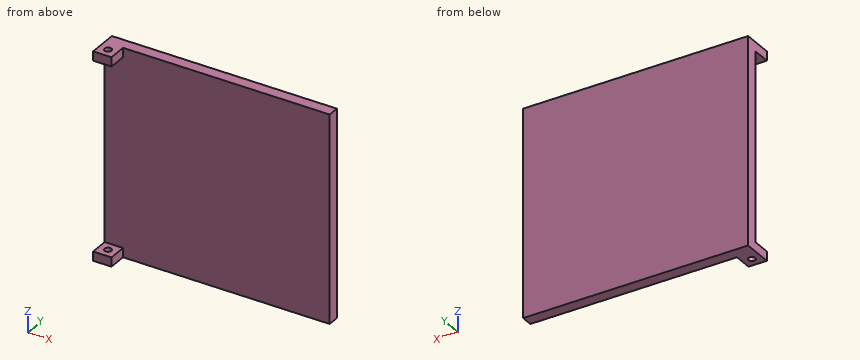
from build123d import *

# Parameters (mm, degrees)
SKETCH_1_W          = 39.2
SKETCH_1_H          = 36
EXTRUDE_1_DEPTH     = 2
SKETCH_7_W          = 3.2
SKETCH_7_H          = 1.6
EXTRUDE_3_DEPTH     = 3.2
CUT_EXTRUDE_START   = -36
SKETCH_8_R          = 0.6
CUT_EXTRUDE_2_DEPTH = 36


with BuildPart() as part:
    # Эскиз1 → Бобышка-Вытянуть1 (new body)
    with BuildSketch(Plane(origin=(0, 0, 0), x_dir=(1, 0, 0), z_dir=(0, 1, 0))):
        Rectangle(SKETCH_1_W, SKETCH_1_H)
    extrude(amount=EXTRUDE_1_DEPTH)

    # Эскиз7 → Бобышка-Вытянуть3 (add)
    with BuildSketch(Plane.XZ):
        with Locations((-18, -17.2)):
            Rectangle(SKETCH_7_W, SKETCH_7_H)
        with Locations((-18, 17.2)):
            Rectangle(SKETCH_7_W, SKETCH_7_H)
    extrude(amount=EXTRUDE_3_DEPTH)

    # Эскиз8 → Вырез-Вытянуть2 (cut)
    with BuildSketch(Plane(origin=(0, 0, -18), x_dir=(-1, 0, 0), z_dir=(0, 0, -1)).offset(CUT_EXTRUDE_START)):
        with Locations((18, -1.6)):
            Circle(SKETCH_8_R)
    extrude(amount=CUT_EXTRUDE_2_DEPTH, mode=Mode.SUBTRACT)


solid = part.part
CAD build for the part. Positions are in the model's coordinates, mm. Round coordinates to 2 decimals unless told otherwise and drop trailing zeros. Write each loop counter-clockwise with the first axis right and the second up, starting at its lowest first coordinate (ties: lowest second). Pieces come first, ordered by that corner, then holes. Notation, with made-up numbers: M 54,13 L 74,13 A20 ccw 74,24 Z; hole C 9,58 d1. An arc over 180 degrees is marked long. Put each result on its own line as item: value. Start each with the question number.
1) Pin check, flat tips, straight feed: pin 1 Ø3 at (x, z) = (6, 7.5) entering from -Y; pin 2 Ø1.8 at (y, z) = (-2, 17) entering from +X; pin 3 Ø1.1 at (x, y) = (-18, -1.6) entering from +Z; pin 4 Ø1.9 at (x, y) = (-18, -1.6) entering from +Z. Stop position of each tip, or through.
2) Saw through at B-B, the plane y = -1.6. Write the cut outline in (x, z).
3) Drill centre lines: probe 1 along Y at (x, z) = (-18, 17); probe 2 along Y at (x, z) = (3, -3); probe 3 along X at (y, z) = (-1.6, 16.9). Where is each one in solid material? Low to high. Write a range as [from, to].
4) Saw through at C-C, the plane z = -7.5. Write the cut outline in (x, y), and give its area (3 significant figures).
5) Saw through at A-A, the plane x = -18. Write the cut outline in (y, z).
6) Saw through at D-D, the plane x = -6. Write the cut outline in (y, z), and give its area (3 significant figures).
Resolved:
1. pin 1: y = 0
1. pin 2: x = -16.4
1. pin 3: through
1. pin 4: z = 18
2. outline: M -19.6,-18 L -18.6,-18 L -18.6,-16.4 L -19.6,-16.4 Z; M -19.6,16.4 L -18.6,16.4 L -18.6,18 L -19.6,18 Z; M -17.4,-18 L -16.4,-18 L -16.4,-16.4 L -17.4,-16.4 Z; M -17.4,16.4 L -16.4,16.4 L -16.4,18 L -17.4,18 Z
3. probe 1: [-3.2, -2.2], [-1, 2]
3. probe 2: [0, 2]
3. probe 3: [-19.6, -18.6], [-17.4, -16.4]
4. outline: M -19.6,0 L 19.6,0 L 19.6,2 L -19.6,2 Z
4. area: 78.4 mm²
5. outline: M -3.2,-18 L -2.2,-18 L -2.2,-16.4 L -3.2,-16.4 Z; M -3.2,16.4 L -2.2,16.4 L -2.2,18 L -3.2,18 Z; M -1,-18 L 2,-18 L 2,18 L -1,18 L -1,16.4 L 0,16.4 L 0,-16.4 L -1,-16.4 Z
6. outline: M 0,-18 L 2,-18 L 2,18 L 0,18 Z
6. area: 72.0 mm²
